Geometry check sheet. Reference: the model listing, model coordinates, mm. Round coordinates to 2 decimals unless told otherwise and drop trailing zeros. Loops run counter-clockwise (first coordinate to the right, second up) from the corner with the lowest first, then second, coordinate; pieces in that order, holes last. Notation, with made-up numbers: (36.25, 32) -> (64.25, 32) arc R33 ccw to (64.25, 71) -> close; hole circle Ø2 at (18, 54.25). An arc over 180 degrees is marked (long way). Use a Markdown table: item, result. Add a question column.
Q1. Sectioned sample at C-C, the plane x = 14.5. Enter the section's corners in (y, z) (3 decimals).
Q2. Sectioned sample at A-A, the plane y = -49.5. Enter the section's corners in (x, z).
Q3. Sectioned sample at D-D, the plane x = 122. Enter the section's corners in (y, z), then the cut area to 3 significant figures.
Q4. Release check for a two-part mould opening along Y. For faces 1 (the face through (-1, 63, 0)), 2 (the face through (-3, -60, 50)), 3 (the face through (-3, 65, 64)), 4 (the face through (-3, 60, 64)) record: released by +Y, released by -Y, zero draft, split by the parting line, or undercut.
Q5. Material ranges on L1, parallel to Y at x = -127, z = 91.5; L2, parallel to Y at x = 26.5, z = 67, recorded low to high.
Q6. Sectioned sample at B-B, the plane z = 114.5. Enter the section's corners in (x, y), then the cut area to 3 significant figures.
```python
from build123d import *

# Parameters (mm, degrees)
SKETCH1_W           = 360
SKETCH1_H           = 130
BOSS_EXTRUDE1_DEPTH = 130
SHELL1_T            = -5
SKETCH2_W           = 350
SKETCH2_H           = 120
CUT_EXTRUDE1_DEPTH  = 232.354706025
SKETCH3_W           = 101.6
SKETCH3_H           = 6.35
CUT_EXTRUDE2_DEPTH  = 255.803846125


with BuildPart() as part:
    # Sketch1 → Boss-Extrude1 (new body)
    with BuildSketch(Plane.XY):
        Rectangle(SKETCH1_W, SKETCH1_H)
    extrude(amount=BOSS_EXTRUDE1_DEPTH)

    # Shell1
    shell1_openings = [part.faces().sort_by_distance(p)[0] for p in [
        (-180, 0, 65),
        (180, 0, 65),
    ]]
    offset(amount=SHELL1_T, openings=shell1_openings, kind=Kind.INTERSECTION)

    # Sketch2 → Cut-Extrude1 (cut, through all)
    with BuildSketch(Plane.XY.offset(130)):
        Rectangle(SKETCH2_W, SKETCH2_H)
    extrude(amount=-CUT_EXTRUDE1_DEPTH, mode=Mode.SUBTRACT)

    # Sketch3 → Cut-Extrude2 (cut, through all)
    with BuildSketch(Plane(origin=(0, -60, 0), x_dir=(1, 0, 0), z_dir=(0, 1, 0))):
        with Locations((0, -65)):
            Rectangle(SKETCH3_W, SKETCH3_H)
    extrude(amount=-CUT_EXTRUDE2_DEPTH, mode=Mode.SUBTRACT)


solid = part.part
```
Values:
| question | item | result |
|---|---|---|
| 1 | outline | (-65, 0) -> (-60, 0) -> (-60, 61.825) -> (-65, 61.825) -> close; (-65, 68.175) -> (-60, 68.175) -> (-60, 130) -> (-65, 130) -> close; (60, 0) -> (65, 0) -> (65, 130) -> (60, 130) -> close |
| 2 | outline | (-180, 0) -> (-175, 0) -> (-175, 5) -> (-180, 5) -> close; (-180, 125) -> (-175, 125) -> (-175, 130) -> (-180, 130) -> close; (175, 0) -> (180, 0) -> (180, 5) -> (175, 5) -> close; (175, 125) -> (180, 125) -> (180, 130) -> (175, 130) -> close |
| 3 | outline | (-65, 0) -> (-60, 0) -> (-60, 130) -> (-65, 130) -> close; (60, 0) -> (65, 0) -> (65, 130) -> (60, 130) -> close |
| 3 | area | 1,300 mm^2 |
| 4 | face 1 | zero draft |
| 4 | face 2 | undercut |
| 4 | face 3 | released by +Y |
| 4 | face 4 | undercut |
| 5 | L1 | -65 to -60, 60 to 65 |
| 5 | L2 | 60 to 65 |
| 6 | outline | (-180, -65) -> (180, -65) -> (180, -60) -> (-180, -60) -> close; (-180, 60) -> (180, 60) -> (180, 65) -> (-180, 65) -> close |
| 6 | area | 3,600 mm^2 |
